from build123d import *

# Parameters (mm, degrees)
F2_DEPTH = 3.175
F3_W     = 76.2
F3_H     = 44.45
F4_DEPTH = 3.175
F6_DEPTH = 3.175


# Not quite as in the source:
# - a variable given as a bare number and used for a length is read in inches; the dataset says mm whatever the document's units were


with BuildPart() as f2:
    # F1 (on Front) → F2 (new body)
    with BuildSketch(Plane.XZ):
        with BuildLine():
            Line((49.53, 120.65), (26.67, 120.65))
            ThreePointArc((26.67, 120.65), (7.8114621458, 112.8385378542), (0, 93.98))
            Line((0, 93.98), (0, 0))
            Line((0, 0), (15.24, 0))
            Line((15.24, 0), (15.24, 93.98))
            ThreePointArc((15.24, 93.98), (18.587769491, 102.062230509), (26.67, 105.41))
            Line((26.67, 105.41), (49.53, 105.41))
            ThreePointArc((49.53, 105.41), (57.612230509, 102.062230509), (60.96, 93.98))
            Line((60.96, 93.98), (60.96, 0))
            Line((60.96, 0), (76.2, 0))
            Line((76.2, 0), (76.2, 93.98))
            ThreePointArc((76.2, 93.98), (68.3885378542, 112.8385378542), (49.53, 120.65))
        make_face()
    extrude(amount=F2_DEPTH)

    # F3 (on Top) → F4 (join)
    with BuildSketch(Plane.XY):
        with Locations((38.1, -22.225)):
            Rectangle(F3_W, F3_H)
    extrude(amount=-F4_DEPTH)

    # F5 (on Front) → F6 (join)
    with BuildSketch(Plane.XZ):
        with BuildLine():
            Line((48.26, 101.6), (27.94, 101.6))
            ThreePointArc((27.94, 101.6), (21.6538207153, 98.9961792847), (19.05, 92.71))
            Line((19.05, 92.71), (19.05, 0))
            Line((19.05, 0), (57.15, 0))
            Line((57.15, 0), (57.15, 92.71))
            ThreePointArc((57.15, 92.71), (54.5461792847, 98.9961792847), (48.26, 101.6))
        make_face()
    extrude(amount=F6_DEPTH)


solid = f2.part
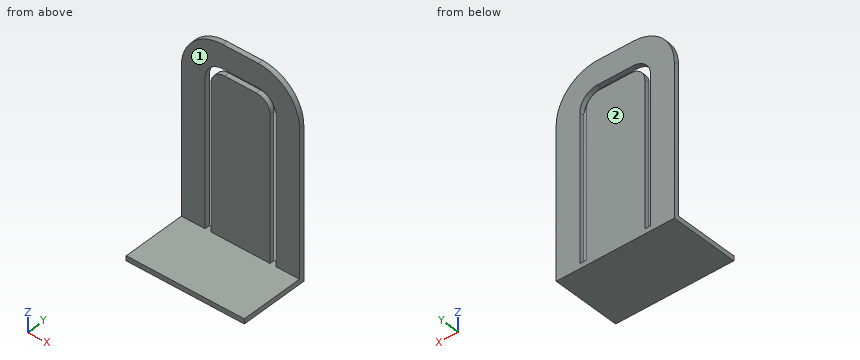
Verification items for the finished model (mm, model axes). Face numbers are marked on the shaded views. A direction names the side the tool comes from. Coordinates: 2 decimals unless noted, no trailing zeros. Order: outer loops, then holes, each group sorted by start corner. A loop starts at its lowest first (then second) coordinate and runs counter-clockwise, first axis right, second up. Notation, with made-up numbers: M -36,-24 L -10,-24 A19 cw -10,-11 Z; hole C -27.5,34.5 d8. An arc over 180 degrees is marked long. One line per item, written item: value. Start each with the question number.
Item 1: Sectioned sample at A-A on x = 42. Record the cut outline in (y, z) (3 decimals).
Item 2: Sectioned sample at D-D on y = -22. Record the cut outline in (x, z) (3 decimals).
Item 3: Depth check by flat-ended pin: P1, Ø1.5, axis at x = 56.5, z = 32, coming from the -Y side (3 decimals); P2, Ø1.5, axis at x = 65.5, z = 62.5, coming from the +Y side. Enter the tip coordinate at first touch or a pass-through.
Item 4: Access from +Z, -Z, +X, -X, +Y, -Y to the whole of each face (thin tool, end or side, straight path). Record for the marked faces 1 and 2.
Item 5: Sectioned sample at C-C on x = 23. Record the cut outline in (y, z) (3 decimals), then the cut area to 3 significant figures.
Item 6: Thickness scan on probe 1 along Z at (x, y) = (33.5, -42) (3 decimals). Record the ranges inside material, lowest first.
Item 7: Sectioned sample at B-B on z = 23. Record the cut outline in (x, y) (3 decimals).
Calculated:
1. outline: M -44.45,-3.175 L 0,-3.175 L 0,101.6 L -3.175,101.6 L -3.175,0 L -44.45,0 Z; M -3.175,105.41 L 0,105.41 L 0,120.65 L -3.175,120.65 Z
2. outline: M 0,-3.175 L 76.2,-3.175 L 76.2,0 L 0,0 Z
3. P1: y = -3.175
3. P2: y = 0
4. face 1: +Z, +X, -X, -Y
4. face 2: +Z, -Z, +X, -X, +Y
5. outline: M -44.45,-3.175 L 0,-3.175 L 0,100.101 L -3.175,100.101 L -3.175,0 L -44.45,0 Z; M -3.175,104.805 L 0,104.805 L 0,120.396 L -3.175,120.396 Z
5. area: 508 mm^2
6. probe 1: -3.175 to 0
7. outline: M 0,-3.175 L 15.24,-3.175 L 15.24,0 L 0,0 Z; M 19.05,-3.175 L 57.15,-3.175 L 57.15,0 L 19.05,0 Z; M 60.96,-3.175 L 76.2,-3.175 L 76.2,0 L 60.96,0 Z
